```python
from build123d import *

# Parameters (mm, degrees)
SKETCH1_W               = 63.5
SKETCH1_H               = 6.35
BOSS_EXTRUDE1_DEPTH     = 126.8095
CUT_EXTRUDE1_DEPTH      = 1
CUT_EXTRUDE1_DEPTH_BACK = 7.35
FILLET1_R               = 12.7
LPATTERN1_COUNT         = 6
LPATTERN1_PITCH         = 22.225


with BuildPart() as part:
    # Sketch1 → Boss-Extrude1 (new body, symmetric)
    with BuildSketch(Plane.XY):
        with Locations((31.75, 3.175)):
            Rectangle(SKETCH1_W, SKETCH1_H)
    extrude(amount=BOSS_EXTRUDE1_DEPTH, both=True)

    # Sketch2 → Cut-Extrude1 (cut, two sides)
    with BuildSketch(Plane(origin=(0, 6.35, 0), x_dir=(1, 0, 0), z_dir=(0, 1, 0))) as cut_extrude1_sk:
        Polygon((-489.189690869, 298.509986386), (0, 120.4595), (38.1, 106.592234074), (38.1, -106.592234074), (0, -120.4595), (-489.189690869, -298.509986386), (-1530.359281964, -298.509986386), (-1530.359281964, 298.509986386), align=None)
    extrude(amount=CUT_EXTRUDE1_DEPTH, mode=Mode.SUBTRACT)
    extrude(cut_extrude1_sk.sketch, amount=-CUT_EXTRUDE1_DEPTH_BACK, mode=Mode.SUBTRACT)

    # Fillet1
    fillet1_edges = [part.edges().sort_by_distance(p)[0] for p in [
        (38.1, 3.175, -106.592234074),
        (38.1, 3.175, 106.592234074),
    ]]
    fillet(fillet1_edges, radius=FILLET1_R)

    # Sketch4 → 5/8 (0.625) Diameter Hole1 (revolve, cut)
    with BuildSketch(Plane(origin=(50.8, 6.35, 0), x_dir=(0, 0, 1), z_dir=(1, 0, 0))):
        Polygon((0, 0), (0, 23.819331164), (7.9375, 19.05), (7.9375, 0), align=None)
    f_5_8_0_625_diameter_hole1 = revolve(axis=Axis((50.8, 12.7, 0), (0, -1, 0)), mode=Mode.SUBTRACT)

    # LPattern1: 5/8 (0.625) Diameter Hole1 ×6
    with Locations(*[(0, 0, -i * LPATTERN1_PITCH) for i in range(1, LPATTERN1_COUNT)]):
        add(f_5_8_0_625_diameter_hole1, mode=Mode.SUBTRACT)

    # Mirror1 copy 1 sketch → Mirror1 copy 1 (revolve, cut)
    with BuildSketch(Plane(origin=(50.8, 6.35, 22.225), x_dir=(0, 0, -1), z_dir=(1, 0, 0))):
        Polygon((0, 0), (0, -23.819331164), (7.9375, -19.05), (7.9375, 0), align=None)
    revolve(axis=Axis((50.8, 12.7, 22.225), (0, 1, 0)), mode=Mode.SUBTRACT)

    # Mirror1 copy 2 sketch → Mirror1 copy 2 (revolve, cut)
    with BuildSketch(Plane(origin=(50.8, 6.35, 44.45), x_dir=(0, 0, -1), z_dir=(1, 0, 0))):
        Polygon((0, 0), (0, -23.819331164), (7.9375, -19.05), (7.9375, 0), align=None)
    revolve(axis=Axis((50.8, 12.7, 44.45), (0, 1, 0)), mode=Mode.SUBTRACT)

    # Mirror1 copy 3 sketch → Mirror1 copy 3 (revolve, cut)
    with BuildSketch(Plane(origin=(50.8, 6.35, 66.675), x_dir=(0, 0, -1), z_dir=(1, 0, 0))):
        Polygon((0, 0), (0, -23.819331164), (7.9375, -19.05), (7.9375, 0), align=None)
    revolve(axis=Axis((50.8, 12.7, 66.675), (0, 1, 0)), mode=Mode.SUBTRACT)

    # Mirror1 copy 4 sketch → Mirror1 copy 4 (revolve, cut)
    with BuildSketch(Plane(origin=(50.8, 6.35, 88.9), x_dir=(0, 0, -1), z_dir=(1, 0, 0))):
        Polygon((0, 0), (0, -23.819331164), (7.9375, -19.05), (7.9375, 0), align=None)
    revolve(axis=Axis((50.8, 12.7, 88.9), (0, 1, 0)), mode=Mode.SUBTRACT)

    # Mirror1 copy 5 sketch → Mirror1 copy 5 (revolve, cut)
    with BuildSketch(Plane(origin=(50.8, 6.35, 111.125), x_dir=(0, 0, -1), z_dir=(1, 0, 0))):
        Polygon((0, 0), (0, -23.819331164), (7.9375, -19.05), (7.9375, 0), align=None)
    revolve(axis=Axis((50.8, 12.7, 111.125), (0, 1, 0)), mode=Mode.SUBTRACT)

    # Mirror1 copy 6 sketch → Mirror1 copy 6 (revolve, cut)
    with BuildSketch(Plane(origin=(50.8, 6.35, 0), x_dir=(0, 0, -1), z_dir=(1, 0, 0))):
        Polygon((0, 0), (0, -23.819331164), (7.9375, -19.05), (7.9375, 0), align=None)
    revolve(axis=Axis((50.8, 12.7, 0), (0, 1, 0)), mode=Mode.SUBTRACT)


solid = part.part
```
Geometry check sheet. Reference: the model listing, model coordinates, mm. A direction names the side the tool comes from. Coordinates: 2 decimals unless noted, no trailing zeros. Write each loop counter-clockwise with the first axis right and the second up, starting at its lowest first coordinate (ties: lowest second). Pieces come first, ordered by that corner, then holes. Notation, with made-up numbers: (64, 0) -> (114, 0) arc R16 ccw to (114, 8) -> close; hole circle Ø6 at (41.5, 63). An arc over 180 degrees is marked (long way). Use CSV: the item, a comma, the result in double quotes. Start each with the question number.
Item 1: Cross-section at B-B, the plane y = 1. State how many separate pieces and enclosed holes the cut face has, plus the area to 3 significant figures.
Item 2: Cross-section at C-C, the plane x = 18. Record the cut outline in (y, z), plus the area to 3 significant figures.
Item 3: Thickness scan on line 1 (X direction, y = 3, z = -88.9); line 2 (Z direction, x = 30, y = 3.25); line 3 (Z direction, x = 5.5, y = 4.25). Record the ranges inside material, lowest first.
Item 4: Mould release check, pull along X, two halves, no side actions. Record for faces 1 (the flat face through (39, 6.35, 1)), 2 (the cylindrical face through (58.549, 3.219, 68.396)), 3 (the flat face through (38.1, 3, -1)), 4 (the cylindrical face through (53.84, 3.219, -59.343)): released by +X, released by -X, zero draft, split by the parting line, or undercut.
Item 5: Cross-section at A-A, the plane z = -88.9. Record the cut outline in (x, y), plus the area to 3 significant figures.
Item 6: Set-up check for faces 5 (the cylindrical face through (35.741, 3.131, -105.073)), 6 (the cylindrical face through (55.63, 3.219, 28.524)): record each of +Z, -Z, +X, -X, +Y, -Y from which the full face is reachable in a straight line by a thin tool's end or side.
Item 7: Depth check by flat-ended pin: pin 1 Ø12.5 at (x, z) = (50.8, 111.125) entering from +Y; pin 2 Ø12 at (x, z) = (48.5, -8) entering from -Y; pin 3 Ø1.9 at (y, z) = (3.5, -17) entering from -X. Enter the tip coordinate at first touch or a pass-through.
Answers:
1,separate pieces,"1"
1,enclosed holes,"11"
1,area,"5,310 mm^2"
2,outline,"(0, -126.81) -> (6.35, -126.81) -> (6.35, -113.91) -> (0, -113.91) -> close; (0, 113.91) -> (6.35, 113.91) -> (6.35, 126.81) -> (0, 126.81) -> close"
2,area,"164 mm^2"
3,line 1,"38.1 to 42.86, 58.74 to 63.5"
3,line 2,"-126.81 to -109.54, 109.54 to 126.81"
3,line 3,"-126.81 to -118.46, 118.46 to 126.81"
4,face 1,"zero draft"
4,face 2,"undercut"
4,face 3,"released by -X"
4,face 4,"undercut"
5,outline,"(38.1, 0) -> (42.86, 0) -> (42.86, 6.35) -> (38.1, 6.35) -> close; (58.74, 0) -> (63.5, 0) -> (63.5, 6.35) -> (58.74, 6.35) -> close"
5,area,"60.5 mm^2"
6,face 5,"-X, +Y, -Y"
6,face 6,"+Y, -Y"
7,pin 1,"through"
7,pin 2,"y = 0"
7,pin 3,"x = 38.1"
